Drawing for the job (mm, zero at the part's lowest x, y, z). A direction names the side the tool comes from. Give positions to 0.01 mm unless a question says otherwise; leave off trailing zeros. Write each loop counter-clockwise with the first axis right and the second up, starting at its lowest first coordinate (ties: lowest second). Pieces come first, ordered by that corner, then holes. Notation, with made-up numbers: (-14, 35.25) - (0, 35.25) arc R23 ccw to (0, 64.25) - close; hole circle Ø11 at (-25.5, -22.75). An arc over 180 degrees is marked (long way). Write item = value, one per line. Start each with the question number.
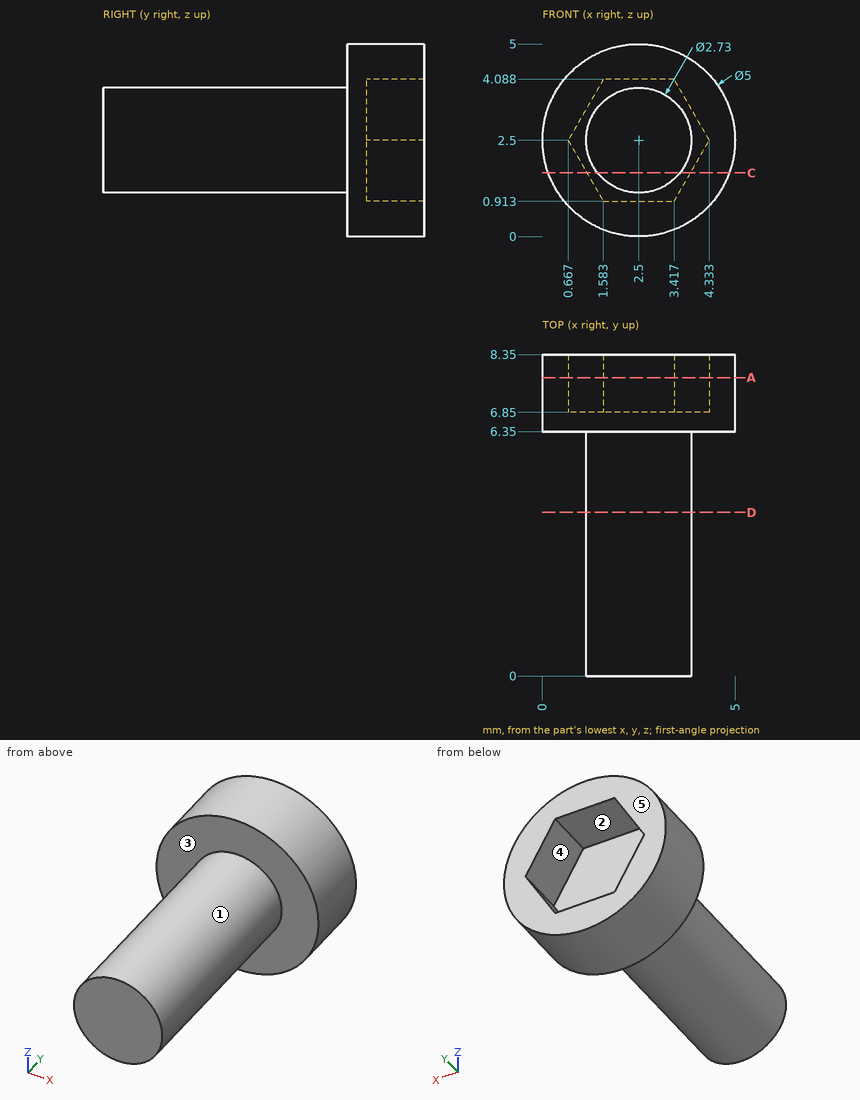
1. Cut at D-D (y = 4.25). Give the cut face in (x, z) (1 decimal).
2. Tool access for the marked faces 4 and 5: list every direction of +Z, -Z, +X, -X, +Y, -Y with a clear straight run to the whole face (end or side of a thin tool).
3. Cut at A-A (y = 7.75). Give the cut face in (x, z).
4. Pin check, flat tips, straight feed: pin 1 Ø3 at (x, y) = (1.5, 5.5) entering from -Z; pin 2 Ø1.5 at (x, z) = (3.5, 0.5) entering from -Y; pin 3 Ø1 at (y, z) = (4, 3.5) entering from +X; pin 4 Ø2 at (x, y) = (4.5, 1.5) entering from +Z. Stop position of each tip, or through.
5. Mould opens along X. For the marked faces 1, 2 and 3 say: +X half, -X half, draft (parallel to the pull), parting line (faces both ways), or undercut.
6. Wall check: line 1 along Y through (x, z) = (3.15, 4.4); line 2 along Y through (x, z) = (3.4, 2.15); line 3 along X through (y, z) = (7, 3.5) (1 decimal). Give the ranges that are in metal, low to high.
7. Cut at C-C (z = 1.65). Give the cut face in (x, y).
Output:
q1.outline = circle Ø2.7 at (2.5, 2.5)
q2.face_4 = +Y
q2.face_5 = +Z, -Z, +X, -X, +Y
q3.outline = circle Ø5 at (2.5, 2.5); hole (0.67, 2.5) - (1.58, 0.91) - (3.42, 0.91) - (4.33, 2.5) - (3.42, 4.09) - (1.58, 4.09) - close
q4.pin_1 = 0
q4.pin_2 = 6.35
q4.pin_3 = 3.77
q4.pin_4 = 3.43
q5.face_1 = parting line
q5.face_2 = undercut
q5.face_3 = draft
q6.line_1 = 6.35 to 8.35
q6.line_2 = 0 to 6.85
q6.line_3 = 0.2 to 1.2, 3.8 to 4.8
q7.outline = (0.15, 6.35) - (1.43, 6.35) - (1.43, 0) - (3.57, 0) - (3.57, 6.35) - (4.85, 6.35) - (4.85, 8.35) - (3.84, 8.35) - (3.84, 6.85) - (1.16, 6.85) - (1.16, 8.35) - (0.15, 8.35) - close
